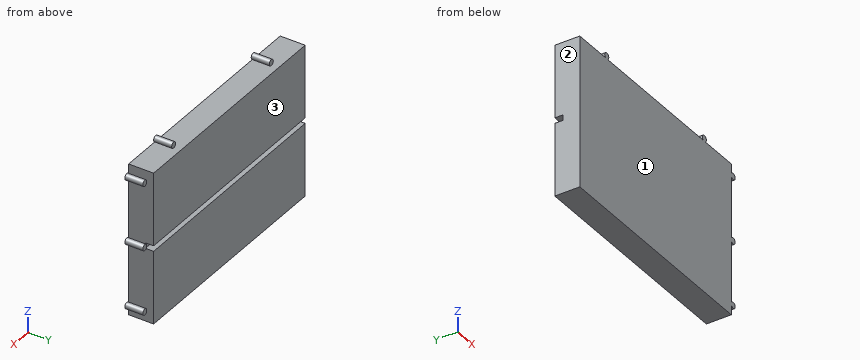
from build123d import *

# Parameters (mm, degrees)
BOSS_EXTRUDE1_DEPTH = 6
SKETCH2_W           = 82.6
SKETCH2_H           = 26.3
BOSS_EXTRUDE2_DEPTH = 3
SKETCH3_W           = 82.6
SKETCH3_H           = 26.3
BOSS_EXTRUDE3_DEPTH = 3
BOSS_EXTRUDE4_DEPTH = 0.5
BOSS_EXTRUDE5_DEPTH = 6.5
BOSS_EXTRUDE6_DEPTH = 6.5
BOSS_EXTRUDE7_DEPTH = 6.5
BOSS_EXTRUDE8_DEPTH = 6.5


with BuildPart() as part:
    # Sketch1 → Boss-Extrude1 (new body)
    with BuildSketch(Plane.XZ):
        with BuildLine():
            Line((-82.6, 0), (0, 0))
            Line((0, 0), (0, 26.841742431))
            ThreePointArc((0, 26.841742431), (2.1, 27.3), (0, 27.758257569))
            Line((0, 27.758257569), (0, 54.6))
            Line((0, 54.6), (-82.6, 54.6))
            Line((-82.6, 54.6), (-82.6, 0))
        make_face()
    extrude(amount=-BOSS_EXTRUDE1_DEPTH)

    # Sketch2 → Boss-Extrude2 (add)
    with BuildSketch(Plane(origin=(0, 6, 0), x_dir=(-1, 0, 0), z_dir=(0, 1, 0))):
        with Locations((41.3, 13.15)):
            Rectangle(SKETCH2_W, SKETCH2_H)
    extrude(amount=BOSS_EXTRUDE2_DEPTH)

    # Sketch3 → Boss-Extrude3 (add)
    with BuildSketch(Plane(origin=(0, 6, 0), x_dir=(-1, 0, 0), z_dir=(0, 1, 0))):
        with Locations((41.3, 41.45)):
            Rectangle(SKETCH3_W, SKETCH3_H)
    extrude(amount=BOSS_EXTRUDE3_DEPTH)

    # Sketch4 → Boss-Extrude4 (add)
    with BuildSketch(Plane(origin=(0, 6, 0), x_dir=(-1, 0, 0), z_dir=(0, 1, 0))):
        with BuildLine():
            Line((0, 27.758257569), (0, 26.841742431))
            ThreePointArc((0, 26.841742431), (-2.1, 27.3), (0, 27.758257569))
        make_face()
    extrude(amount=BOSS_EXTRUDE4_DEPTH)

    # Sketch5 → Boss-Extrude5 (add)
    with BuildSketch(Plane.XZ):
        with BuildLine():
            Line((0, 4.458257629), (0, 3.54174249))
            ThreePointArc((0, 3.54174249), (2.1, 4.00000006), (0, 4.458257629))
        make_face()
    extrude(amount=-BOSS_EXTRUDE5_DEPTH)

    # Sketch6 → Boss-Extrude6 (add)
    with BuildSketch(Plane.XZ):
        with BuildLine():
            Line((0, 51.05825751), (0, 50.141742371))
            ThreePointArc((0, 50.141742371), (2.1, 50.59999994), (0, 51.05825751))
        make_face()
    extrude(amount=-BOSS_EXTRUDE6_DEPTH)

    # Sketch7 → Boss-Extrude7 (add)
    with BuildSketch(Plane.XZ):
        with BuildLine():
            Line((-68.358257569, 54.6), (-67.441742431, 54.6))
            ThreePointArc((-67.441742431, 54.6), (-67.9, 56.7), (-68.358257569, 54.6))
        make_face()
    extrude(amount=-BOSS_EXTRUDE7_DEPTH)

    # Sketch8 → Boss-Extrude8 (add)
    with BuildSketch(Plane.XZ):
        with BuildLine():
            Line((-15.158257569, 54.6), (-14.241742431, 54.6))
            ThreePointArc((-14.241742431, 54.6), (-14.7, 56.7), (-15.158257569, 54.6))
        make_face()
    extrude(amount=-BOSS_EXTRUDE8_DEPTH)


solid = part.part
Source: CAD feature listing. Evaluate the final solid. Frame: model axes, mm. Face numbers are marked on the shaded views. Give positions to 0.01 mm unless a question says otherwise; leave off trailing zeros. Order: outer loops, then holes, each group sorted by start corner. A loop starts at its lowest first (then second) coordinate and runs counter-clockwise, first axis right, second up. Notation, with made-up numbers: (29, 16) -> (42, 16) arc R15 ccw to (42, 20) -> close; hole circle Ø4 at (64, 7.25). An arc over 180 degrees is marked (long way). Use a Markdown table: item, result.
1) Ray query, line 1 along Z through (x, y) = (-53.5, 7.25); line 2 along X through (y, z) = (7.5, 24); line 3 along Z through (x, y) = (-66.5, 3.25). Return the intervals inside material, ascending. Write a range as [from, to].
Answer list:
| item | result |
|---|---|
| line 1 | [0, 26.3], [28.3, 54.6] |
| line 2 | [-82.6, 0] |
| line 3 | [0, 54.6] |
2) Section query C-C, the plane x = -42.5. Return the cut outline in (y, z), then the cut area to 3 significant figures.
Answer list:
| item | result |
|---|---|
| outline | (0, 0) -> (9, 0) -> (9, 26.3) -> (6, 26.3) -> (6, 28.3) -> (9, 28.3) -> (9, 54.6) -> (0, 54.6) -> close |
| area | 485 mm² |
3) Section query A-A, the plane x = 1. Return the cut outline in (y, z), then the cut area to 3 significant figures.
Answer list:
| item | result |
|---|---|
| outline | (0, 2.9) -> (6.5, 2.9) -> (6.5, 5.1) -> (0, 5.1) -> close; (0, 26.2) -> (6.5, 26.2) -> (6.5, 28.4) -> (0, 28.4) -> close; (0, 49.5) -> (6.5, 49.5) -> (6.5, 51.7) -> (0, 51.7) -> close |
| area | 42.9 mm² |
4) Mould query, pull axis Y, two halves, no side actions, for the marked faces 1, 2 and 3. Classes: +Y half, -Y half, draft (parallel to the pull), parting line (faces both ways), or undercut.
Answer list:
| item | result |
|---|---|
| face 1 | -Y half |
| face 2 | draft |
| face 3 | +Y half |
5) Section query B-B, the plane z = 55.6. Return the cut outline in (x, y).
Answer list:
| item | result |
|---|---|
| outline | (-69, 0) -> (-66.8, 0) -> (-66.8, 6.5) -> (-69, 6.5) -> close; (-15.8, 0) -> (-13.6, 0) -> (-13.6, 6.5) -> (-15.8, 6.5) -> close |
6) Section query D-D, the plane y = 4.75. Return the cut outline in (x, z), then the cut area to 3 significant figures.
Answer list:
| item | result |
|---|---|
| outline | (-82.6, 0) -> (0, 0) -> (0, 3.54) arc R1.1 ccw (long way) to (0, 4.46) -> (0, 26.84) arc R1.1 ccw (long way) to (0, 27.76) -> (0, 50.14) arc R1.1 ccw (long way) to (0, 51.06) -> (0, 54.6) -> (-14.24, 54.6) arc R1.1 ccw (long way) to (-15.16, 54.6) -> (-67.44, 54.6) arc R1.1 ccw (long way) to (-68.36, 54.6) -> (-82.6, 54.6) -> close |
| area | 4,530 mm² |
7) Contact query for flat-ended pins moving along their axis: P1, Ø1.7, axis at x = -15, z = 56, coming from the +Y side; P2, Ø2.5, axis at y = 5.5, z = 19, coming from the +X side; P3, Ø0.9, axis at x = -21.5, y = 7.5, coming from the +Z side. Output: stop coordinate, or through.
Answer list:
| item | result |
|---|---|
| P1 | y = 6.5 |
| P2 | x = 0 |
| P3 | z = 54.6 |
